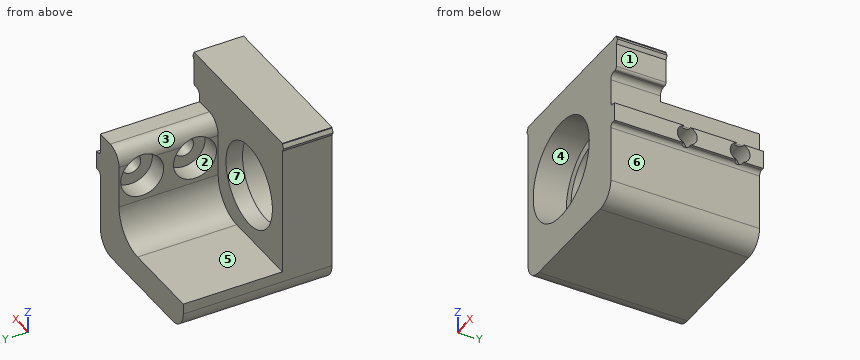
from build123d import *

# Parameters (mm, degrees)
F1_DEPTH  = 55
F3_DEPTH  = 30
F4_R      = 3
F5_DEPTH  = 25
F6_R      = 12.5
F7_DEPTH  = 55.0010001
F8_R      = 15.1
F9_DEPTH  = 20
F10_R     = 6.5
F11_DEPTH = 17
F12_R     = 10
F13_W     = 62.573639676
F13_H     = 57.5273763388
F14_DEPTH = 10


# Not quite as in the source:
# - a feature names something its author has since deleted; it is built from what else it names


with BuildPart() as f1:
    # F0 (on Front) → F1 (new body)
    with BuildSketch(Plane.XZ):
        with BuildLine():
            Line((-23.6999987811, 23.7999986857), (-23.6999987811, 23.5588453133))
            Line((-23.6999987811, 23.5588453133), (-24.3690585991, 22.3999992996))
            Line((-24.3690585991, 22.3999992996), (-23.6999987811, 21.241153286))
            Line((-23.6999987811, 21.241153286), (-23.6999987811, -21.0000007004))
            ThreePointArc((-23.6999987811, -21.0000007004), (-22.0012182918, -25.1012195971), (-17.899999395, -26.8000000864))
            Line((-17.899999395, -26.8000000864), (15.100000605, -26.8000000864))
            ThreePointArc((15.100000605, -26.8000000864), (19.2012195018, -25.1012195971), (20.8999999911, -21.0000007004))
            Line((20.8999999911, -21.0000007004), (20.8999999911, -4.0000007004))
            ThreePointArc((20.8999999911, -4.0000007004), (21.2514720335, -3.1514721288), (22.100000605, -2.8000000864))
            Line((22.100000605, -2.8000000864), (22.8999999911, -2.8000000864))
            Line((22.8999999911, -2.8000000864), (22.8999999911, 2.7999986857))
            Line((22.8999999911, 2.7999986857), (22.100000605, 2.7999986857))
            ThreePointArc((22.100000605, 2.7999986857), (21.2514720335, 3.1514707281), (20.8999999911, 3.9999992996))
            Line((20.8999999911, 3.9999992996), (20.8999999911, 11.4999992996))
            ThreePointArc((20.8999999911, 11.4999992996), (21.3979186429, 12.7020812618), (22.600000605, 13.1999999136))
            Line((22.600000605, 13.1999999136), (23.100000605, 13.1999999136))
            ThreePointArc((23.100000605, 13.1999999136), (23.6656855958, 13.4343143088), (23.8999999911, 13.9999992996))
            Line((23.8999999911, 13.9999992996), (23.8999999911, 21.241153286))
            Line((23.8999999911, 21.241153286), (24.5690598091, 22.3999992996))
            Line((24.5690598091, 22.3999992996), (23.8999999911, 23.5588453133))
            Line((23.8999999911, 23.5588453133), (23.8999999911, 23.7999986857))
            Line((23.8999999911, 23.7999986857), (-23.6999987811, 23.7999986857))
        make_face()
    extrude(amount=F1_DEPTH)

    # F2 (on face) → F3 (cut)
    with BuildSketch(Plane(origin=(0, 0, 0), x_dir=(-1, 0, 0), z_dir=(0, 1, 0))):
        with BuildLine():
            Line((-9.7267732358, -17.8000000864), (27.0197465134, -17.8000000864))
            Line((27.0197465134, -17.8000000864), (27.0197465134, 29.101931586))
            Line((27.0197465134, 29.101931586), (-25.6962114531, 29.101931586))
            Line((-25.6962114531, 29.101931586), (-25.6962114531, 9.6292318066))
            Line((-25.6962114531, 9.6292318066), (-15.5874993246, 9.6292318066))
            ThreePointArc((-15.5874993246, 9.6292318066), (-12.272936759, 8.2562950386), (-10.8999999911, 4.9417324731))
            Line((-10.8999999911, 4.9417324731), (-10.8999999911, -12.1750008862))
            Line((-10.8999999911, -12.1750008862), (-10.8999999911, -17.8000000864))
            Line((-10.8999999911, -17.8000000864), (-9.7267732358, -17.8000000864))
        make_face()
    extrude(amount=-F3_DEPTH, mode=Mode.SUBTRACT)

    # F4 (on face) → F5 (cut)
    with BuildSketch(Plane.YZ.offset(22.8999999911)):
        with Locations((-7, -1.3143e-06)):
            Circle(F4_R)
        with Locations((-23, -1.3143e-06)):
            Circle(F4_R)
    extrude(amount=-F5_DEPTH, mode=Mode.SUBTRACT)

    # F6 (on face) → F7 (cut, through all)
    with BuildSketch(Plane(origin=(0, 0, 0), x_dir=(-1, 0, 0), z_dir=(0, 1, 0))):
        with Locations((5.7999987811, -0.9000000864)):
            Circle(F6_R)
    extrude(amount=-F7_DEPTH, mode=Mode.SUBTRACT)

    # F8 (on face) → F9 (cut)
    with BuildSketch(Plane.XZ.offset(55)):
        with Locations((-5.7999987811, -0.9000000864)):
            Circle(F8_R)
    extrude(amount=-F9_DEPTH, mode=Mode.SUBTRACT)

    # F10 (on Right) → F11 (cut)
    with BuildSketch(Plane.YZ):
        with Locations((-23, 0)):
            Circle(F10_R)
        with Locations((-7, 0)):
            Circle(F10_R)
    extrude(amount=F11_DEPTH, mode=Mode.SUBTRACT)

    # F12
    f12_edges = [f1.edges().sort_by_distance(p)[0] for p in [
        (10.9, -15, -17.8),
    ]]
    fillet(f12_edges, radius=F12_R)

    # F13 (on face) → F14 (cut)
    with BuildSketch(Plane.XZ.offset(55)):
        with Locations((1.9923495129, 0.0138776377)):
            Rectangle(F13_W, F13_H)
    extrude(amount=-F14_DEPTH, mode=Mode.SUBTRACT)


solid = f1.part
Can you work these out from the model? Positions are in its coordinate system, mm. Face numbers are marked on the shaded views. A direction names the side the tool comes from. Coordinates: 2 decimals unless noted, no trailing zeros. Loops run counter-clockwise (first coordinate to the right, second up) from the corner with the lowest first, then second, coordinate; pieces in that order, holes last. Notation, with made-up numbers: (82, 81.25) - (123, 81.25) arc R11 cw to (123, 93.25) - close; hole circle Ø9 at (-20.75, -23). An arc over 180 degrees is marked (long way). Answer as a JSON object with one key per item and string values. Group by question number.
Item 1: If we section it at D-D (z = -20): List the corners of the cut face in (x, y) for me.
Item 2: If I drill on L1, parallel to Y at x = 16, z = 0; L2, parallel to X at y = -19, z = 0.5; L3, parallel to Z at x = 16, y = -18.5, over which ranges is the centre line in solid material (lowest first)? Write a range as from..to.
Item 3: For pin 1 (2 mm diameter, centred on y = -34, z = 18.5, fed in from +X); pin 2 (6 mm diameter, centred on y = -11, z = -10, fed in from +X); pin 3 (10.5 mm diameter, centred on y = -21, z = -2.5, fed in from -X), each with a flat end and sliding along its axis, tell me the tip position at first contact or that it passes through.
Item 4: On a 3-axis mill with a long thin cutter (end or side, diameter ignored), from which of +Z, -Z, +X, -X, +Y, -Y can I reach the whole of each face in a straight line? I mean the marked faces 1, 2, 3 and 4. Say none if no direction works.
Item 5: If we mould it in two halves opening along X, with no side actions, what happens to the marked faces 5, 6 and 7? For each: released by +X, released by -X, zero draft, split by the parting line, or undercut.
Item 6: If we section it at B-B (x = -16): List the corners of the cut face in (y, z) for me.
Item 7: If we section it at C-C (y = -7): List the corners of the cut face in (x, z) for me (1 decimal), plus the area to 3 significant figures.
Item 8: If we section it at A-A (y = -40.5): List the corners of the cut face in (x, z) for me.
Returned:
{
 "1": {"outline": "(-23.7, -45) - (20.9, -45) - (20.9, 0) - (-23.7, 0) - close"},
 "2": {"L1": "y = -45..-29.5, -16.5..-13.5, -0.5..0", "L2": "x = 17..22.9", "L3": "z = -26.73..-4.69, 4.69..9.63"},
 "3": {"pin 1": "stops at x = 23.9", "pin 2": "stops at x = 20.9", "pin 3": "stops at x = 10.9"},
 "4": {"face 1": "-Z, +X, +Y, -Y", "face 2": "-X", "face 3": "+Z, -X, +Y", "face 4": "-Y"},
 "5": {"face 5": "zero draft", "face 6": "released by +X", "face 7": "undercut"},
 "6": {"outline": "(-45, -26.8) - (0, -26.8) - (0, -17.8) - (-30, -17.8) - (-30, -8.13) - (-35, -8.13) - (-35, -12.03) - (-45, -12.03) - close; (-45, 10.23) - (-35, 10.23) - (-35, 6.33) - (-30, 6.33) - (-30, 23.8) - (-45, 23.8) - close"},
 "7": {"outline": "(-23.7, -21) arc R5.8 ccw to (-17.9, -26.8) - (15.1, -26.8) arc R5.8 ccw to (20.9, -21) - (20.9, -4) arc R1.2 cw to (21.4, -3) - (17, -3) - (17, -6.5) - (10.9, -6.5) - (10.9, -7.8) arc R10 cw to (0.9, -17.8) - (-23.7, -17.8) - close; (11.2, 6.5) - (17, 6.5) - (17, 3) - (21.4, 3) arc R1.2 cw to (20.9, 4) - (20.9, 9.6) - (15.6, 9.6) arc R4.7 ccw to start", "area": "576 mm²"},
 "8": {"outline": "(-24.37, 22.4) - (-23.7, 21.24) - (-23.7, -21) arc R5.8 ccw to (-17.9, -26.8) - (15.1, -26.8) arc R5.8 ccw to (20.9, -21) - (20.9, -4) arc R1.2 cw to (22.1, -2.8) - (22.9, -2.8) - (22.9, 2.8) - (22.1, 2.8) arc R1.2 cw to (20.9, 4) - (20.9, 11.5) arc R1.7 cw to (22.6, 13.2) - (23.1, 13.2) arc R0.8 ccw to (23.9, 14) - (23.9, 21.24) - (24.57, 22.4) - (23.9, 23.56) - (23.9, 23.8) - (-23.7, 23.8) - (-23.7, 23.56) - close; hole circle Ø30.2 at (-5.8, -0.9)"}
}
